Geometry: final body of the model. Coordinates: model frame, mm. Face numbers are marked on the shaded views. A direction names the side the tool comes from. Round coordinates to 2 decimals unless told otherwise and drop trailing zeros. Order: outer loops, then holes, each group sorted by start corner. A loop starts at its lowest first (then second) coordinate and runs counter-clockwise, first axis right, second up. Notation, with made-up numbers: M 11.25,38.5 L 45.25,38.5 A19 ccw 45.25,44.5 Z; hole C -37.5,85.25 d7. An arc over 180 degrees is marked long. Return JSON: item names as keys, results as strings. Group by question number.
Q1. Cut plane A-A on z = 85. Output: boundary loops of the cut face in (x, y), and give its area (3 significant figures).
Q2. Access query for the marked faces 4 and 5. Directions: +Z, -Z, +X, -X, +Y, -Y. A direction counts if a zero-diameter tool reaches every point of the face in a straight line with its end or side. Return the directions, or none.
Q3. Cut plane D-D on z = 37. Output: boundary loops of the cut face in (x, y), and give its area (3 significant figures).
Q4. Ray query, probe 1 along X at (y, z) = (-15, 49); probe 2 along X at (y, z) = (33.9, 85). Return the intervals inside material, ascending.
Q5. Cut plane C-C on x = 0. Output: boundary loops of the cut face in (y, z).
Q6. Contact query for flat-ended pins moving along their axis: pin 1 (1 mm diameter, centred on y = 33.5, z = 85.5, fed in from -X); pin 2 (0.6 mm diameter, centred on y = 33.5, z = 87, fed in from +X); pin 3 (25 mm diameter, centred on x = -1.5, z = 71, fed in from -Y). Output: stop coordinate, or through.
Q7. Mould query, pull axis Y, two halves, no side actions, for the marked faces 1, 2 and 3. Classes: released by +Y, released by -Y, zero draft, split by the parting line, or undercut.
Q8. Cut plane B-B on y = 18.5. Output: boundary loops of the cut face in (x, z), and give its area (3 significant figures).
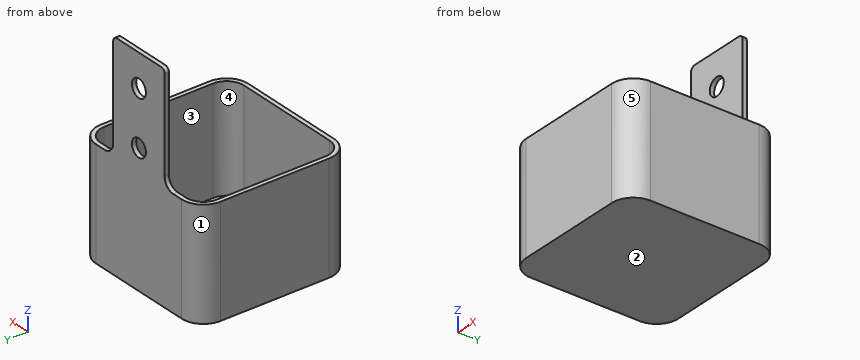
```python
from build123d import *

# Parameters (mm, degrees)
SKETCH1_W           = 70
SKETCH1_H           = 70
BOSS_EXTRUDE1_DEPTH = 50
FILLET1_R           = 10
SHELL1_T            = -2
SKETCH2_W           = 30
SKETCH2_H           = 50
SKETCH2_R           = 4.1
BOSS_EXTRUDE2_DEPTH = 2
FILLET2_R           = 5
FILLET3_R           = 2


with BuildPart() as part:
    # Sketch1 → Boss-Extrude1 (new body)
    with BuildSketch(Plane.XY):
        Rectangle(SKETCH1_W, SKETCH1_H)
    extrude(amount=BOSS_EXTRUDE1_DEPTH)

    # Fillet1
    fillet1_edges = [part.edges().sort_by_distance(p)[0] for p in [
        (35, -35, 25),
        (-35, -35, 25),
        (-35, 35, 25),
        (35, 35, 25),
    ]]
    fillet(fillet1_edges, radius=FILLET1_R)

    # Shell1
    shell1_openings = [part.faces().sort_by_distance(p)[0] for p in [
        (0, 0, 50),
    ]]
    offset(amount=SHELL1_T, openings=shell1_openings, kind=Kind.INTERSECTION)

    # Sketch2 → Boss-Extrude2 (add)
    with BuildSketch(Plane(origin=(0, 35, 0), x_dir=(1, 0, 0), z_dir=(0, 1, 0))):
        with Locations((0, -75)):
            Rectangle(SKETCH2_W, SKETCH2_H)
        with Locations(Location((0, -85, 0), (0, 0, 270))):
            Circle(SKETCH2_R, mode=Mode.SUBTRACT)
        with Locations(Location((0, -60, 0), (0, 0, 270))):
            Circle(SKETCH2_R, mode=Mode.SUBTRACT)
    extrude(amount=-BOSS_EXTRUDE2_DEPTH)

    # Fillet2
    fillet2_edges = [part.edges().sort_by_distance(p)[0] for p in [
        (15, 34, 50),
        (-15, 34, 50),
    ]]
    fillet(fillet2_edges, radius=FILLET2_R)

    # Fillet3
    fillet3_edges = [part.edges().sort_by_distance(p)[0] for p in [
        (-15, 34, 100),
        (15, 34, 100),
    ]]
    fillet(fillet3_edges, radius=FILLET3_R)


solid = part.part
```
Result sheet:
{
 "1": {"outline": "M -15,33 L -4.1,33 L -4.1,35 L -15,35 Z; M 4.1,33 L 15,33 L 15,35 L 4.1,35 Z", "area": "43.6 mm²"},
 "2": {"face 4": "+Z", "face 5": "+Z, -Z, +X, -Y"},
 "3": {"outline": "M -35,-25 A10 ccw -25,-35 L 25,-35 A10 ccw 35,-25 L 35,25 A10 ccw 25,35 L -25,35 A10 ccw -35,25 Z; hole M -33,-25 A8 ccw -25,-33 L 25,-33 A8 ccw 33,-25 L 33,25 A8 ccw 25,33 L -25,33 A8 ccw -33,25 Z", "area": "513 mm²"},
 "4": {"probe 1": "x = -35 to -33, 33 to 35", "probe 2": "x = -15 to -4.1, 4.1 to 15"},
 "5": {"outline": "M -35,0 L 35,0 L 35,55.9 L 33,55.9 L 33,2 L -33,2 L -33,50 L -35,50 Z; M 33,64.1 L 35,64.1 L 35,80.9 L 33,80.9 Z; M 33,89.1 L 35,89.1 L 35,100 L 33,100 Z"},
 "6": {"pin 1": "stops at x = -15", "pin 2": "stops at x = 15", "pin 3": "stops at y = 33"},
 "7": {"face 1": "released by +Y", "face 2": "zero draft", "face 3": "undercut"},
 "8": {"outline": "M -35,0 L 35,0 L 35,50 L 33,50 L 33,2 L -33,2 L -33,50 L -35,50 Z", "area": "332 mm²"}
}
